```python
from build123d import *

# Parameters (mm, degrees)
SKETCH_1_W      = 35
SKETCH_1_H      = 80
EXTRUDE_1_DEPTH = 5
EXTRUDE_2_DEPTH = 45
FILLET_1_R      = 3


with BuildPart() as part:
    # 草圖1 → 填料-伸長1 (new body)
    with BuildSketch(Plane.XY):
        with Locations((-18.303993018, -26.708112773)):
            Rectangle(SKETCH_1_W, SKETCH_1_H)
    extrude(amount=EXTRUDE_1_DEPTH)

    # 草圖3 → 填料-伸長2 (add)
    with BuildSketch(Plane.XY.offset(5)):
        Polygon((-35.803993018, 13.291887227), (-35.803993018, -66.708112773), (-0.803993018, -66.708112773), (-0.803993018, -61.708112773), (-30.803993018, -61.708112773), (-30.803993018, 8.291887227), (-0.803993018, 8.291887227), (-0.803993018, 13.291887227), align=None)
    extrude(amount=EXTRUDE_2_DEPTH)

    # 圓角1
    fillet_1_edges = [part.edges().sort_by_distance(p)[0] for p in [
        (-0.803993018, -64.208112773, 50),
        (-0.803993018, 10.791887227, 50),
    ]]
    fillet(fillet_1_edges, radius=FILLET_1_R)


solid = part.part
```
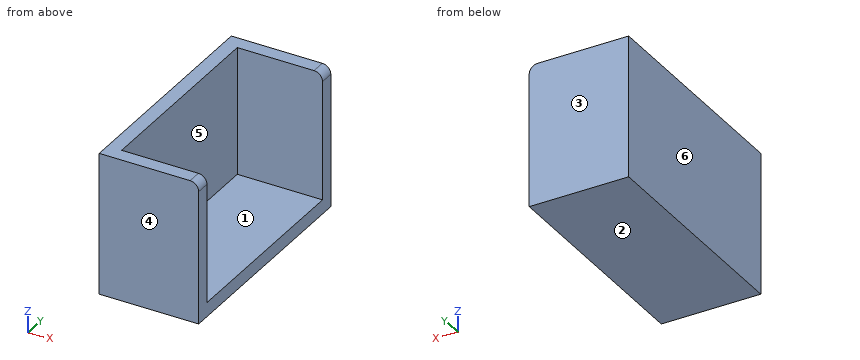
The listing builds one solid part. Answer for the finished solid, in the listing's coordinates (mm). Face numbers are marked on the shaded views. A direction names the side the tool comes from. Coordinates: 2 decimals unless noted, no trailing zeros. Write each loop counter-clockwise with the first axis right and the second up, starting at its lowest first coordinate (ties: lowest second). Pieces come first, ordered by that corner, then holes. Notation, with made-up numbers: (84, 0.25) - (103, 0.25) arc R11 cw to (103, 5.25) - close; hole circle Ø8 at (-14.75, 65). An arc over 180 degrees is marked (long way). One line per item, written item: value.
1) Each of these flat-tipped pins is pushed along its axis until it touches: pin 1 Ø1 at (y, z) = (-12, 30) entering from +X; pin 2 Ø9 at (x, y) = (-11.5, -11) entering from +Z. Where does it stop, or does it pass through?
Geometry check:
pin 1: stops at x = -30.8
pin 2: stops at z = 5
2) For a pull along Y with two mould halves and no side action, classify the marked faces 1, 2, 3 and 4 as pulls with the +Y half, pulls with the -Y half, needs draft (parallel to the pull), parting line crosses it, or undercut.
Geometry check:
face 1: undercut
face 2: needs draft
face 3: pulls with the +Y half
face 4: pulls with the -Y half
3) A tool of negligible diameter and unlimited length cuts with its end or side. For the marked faces 5 and 6, from which of +Z, -Z, +X, -X, +Y, -Y can it reach the whole face along a straight path? Write none if from no direction.
Geometry check:
face 5: +Z, +X
face 6: +Z, -Z, -X, +Y, -Y
4) Find section A-A (z = 21). Give the vertices of the cut face in (x, y).
Geometry check:
outline: (-35.8, -66.71) - (-0.8, -66.71) - (-0.8, -61.71) - (-30.8, -61.71) - (-30.8, 8.29) - (-0.8, 8.29) - (-0.8, 13.29) - (-35.8, 13.29) - close
5) Find section C-C (y = -38.5). Give the vertices of the cut face in (x, z).
Geometry check:
outline: (-35.8, 0) - (-0.8, 0) - (-0.8, 5) - (-30.8, 5) - (-30.8, 50) - (-35.8, 50) - close
6) Consider line 1 along Y through (x, z) = (-23, 40.5); line 2 along X through (y, z) = (-31, 25); line 3 along Z through (x, y) = (-24, -42.5). Determine where each line is inside the solid, lowest interval first. Write a range as from..to.
Geometry check:
line 1: y = -66.71..-61.71, 8.29..13.29
line 2: x = -35.8..-30.8
line 3: z = 0..5
7) Find section B-B (x = -20). Give the vertices of the cut face in (y, z), and give its area (3 significant figures).
Geometry check:
outline: (-66.71, 0) - (13.29, 0) - (13.29, 50) - (8.29, 50) - (8.29, 5) - (-61.71, 5) - (-61.71, 50) - (-66.71, 50) - close
area: 850 mm2
